```python
from build123d import *

# Parameters (mm, degrees)
EXTRUDE1_DEPTH     = 3.81
EXTRUDE2_DEPTH     = 0.508
CUT_EXTRUDE2_DEPTH = 15.094711526
EXTRUDE3_DEPTH     = 3.048
EXTRUDE4_REACH     = 14.678
SKETCH9_W          = 3.045663376
SKETCH9_H          = 0.1905
SKETCH11_R         = 2.286
CUT_EXTRUDE3_DEPTH = 13.677755519
SKETCH12_R         = 3.175
CUT_EXTRUDE4_DEPTH = 0.508
SKETCH13_OUTSIDE_W = 29.435
SKETCH13_OUTSIDE_H = 14.576
SKETCH13_OUTSIDE_R = 3.81
CUT_EXTRUDE5_DEPTH = 15.094711526
CUT_EXTRUDE7_START = 6.096
CUT_EXTRUDE7_DEPTH = 6.096


with BuildPart() as part:
    # Sketch1 → Extrude1 (new body)
    with BuildSketch(Plane(origin=(0, 0, 0), x_dir=(1, 0, 0), z_dir=(0, 1, 0))):
        with BuildLine():
            Line((-8.001, 3.556), (0, 3.556))
            ThreePointArc((0, 3.556), (3.556, 0), (0, -3.556))
            Line((0, -3.556), (-8.001, -3.556))
            ThreePointArc((-8.001, -3.556), (-11.557, 0), (-8.001, 3.556))
        make_face()
    extrude(amount=EXTRUDE1_DEPTH)

    # Sketch4 → Extrude2 (add)
    with BuildSketch(Plane.XY.offset(3.556)):
        with BuildLine():
            Line((0, 0), (0, 3.81))
            Line((0, 3.81), (7.112, 3.81))
            ThreePointArc((7.112, 3.81), (9.806076836, 2.694076836), (10.922, 0))
            Line((10.922, 0), (7.112, 0))
            Line((7.112, 0), (0, 0))
        make_face()
    extrude2 = extrude(amount=-EXTRUDE2_DEPTH)

    # Sketch6 → Cut-Extrude2 (cut, through all)
    with BuildSketch(Plane.XY.offset(3.556)):
        with BuildLine():
            Line((6.35, 2.032), (6.35, 1.016))
            ThreePointArc((6.35, 1.016), (6.275605122, 0.836394878), (6.096, 0.762))
            Line((6.096, 0.762), (5.08, 0.762))
            ThreePointArc((5.08, 0.762), (4.900394878, 0.687605122), (4.826, 0.508))
            Line((4.826, 0.508), (4.826, -0.508))
            ThreePointArc((4.826, -0.508), (4.900394878, -0.687605122), (5.08, -0.762))
            Line((5.08, -0.762), (6.096, -0.762))
            ThreePointArc((6.096, -0.762), (6.275605122, -0.836394878), (6.35, -1.016))
            Line((6.35, -1.016), (6.35, -2.032))
            ThreePointArc((6.35, -2.032), (6.424394878, -2.211605122), (6.604, -2.286))
            Line((6.604, -2.286), (7.62, -2.286))
            ThreePointArc((7.62, -2.286), (7.799605122, -2.211605122), (7.874, -2.032))
            Line((7.874, -2.032), (7.874, -1.016))
            ThreePointArc((7.874, -1.016), (7.948394878, -0.836394878), (8.128, -0.762))
            Line((8.128, -0.762), (9.144, -0.762))
            ThreePointArc((9.144, -0.762), (9.323605122, -0.687605122), (9.398, -0.508))
            Line((9.398, -0.508), (9.398, 0.508))
            ThreePointArc((9.398, 0.508), (9.323605122, 0.687605122), (9.144, 0.762))
            Line((9.144, 0.762), (8.128, 0.762))
            ThreePointArc((8.128, 0.762), (7.948394878, 0.836394878), (7.874, 1.016))
            Line((7.874, 1.016), (7.874, 2.032))
            ThreePointArc((7.874, 2.032), (7.799605122, 2.211605122), (7.62, 2.286))
            Line((7.62, 2.286), (6.604, 2.286))
            ThreePointArc((6.604, 2.286), (6.424394878, 2.211605122), (6.35, 2.032))
        make_face()
    cut_extrude2 = extrude(amount=-CUT_EXTRUDE2_DEPTH, mode=Mode.SUBTRACT)

    # Sketch8 → Extrude3 (add)
    with BuildSketch(Plane(origin=(0, 0, 3.048), x_dir=(-1, 0, 0), z_dir=(0, 0, -1))):
        with BuildLine():
            Line((-10.287, 0), (-9.906, 0))
            ThreePointArc((-9.906, 0), (-9.218056742, 1.836017701), (-7.493, 2.767900829))
            Line((-7.493, 2.767900829), (-7.493, 3.152057106))
            ThreePointArc((-7.493, 3.152057106), (-9.487952441, 2.106056742), (-10.287, 0))
        make_face()
        with BuildLine():
            Line((-4.318, 0), (-3.937, 0))
            ThreePointArc((-3.937, 0), (-4.736047559, 2.106056742), (-6.731, 3.152057106))
            Line((-6.731, 3.152057106), (-6.731, 2.767900829))
            ThreePointArc((-6.731, 2.767900829), (-5.005943258, 1.836017701), (-4.318, 0))
        make_face()
    extrude3 = extrude(amount=EXTRUDE3_DEPTH)

    # Sketch9 → Extrude4 (add, up to next)
    with BuildSketch(Plane(origin=(0, 0, 0), x_dir=(-1, 0, 0), z_dir=(0, 0, -1)), mode=Mode.PRIVATE) as extrude4_sk1:
        with Locations((-2.604668312, 0.09525)):
            Rectangle(SKETCH9_W, SKETCH9_H)
    extrude4_tool1 = extrude(extrude4_sk1.sketch, amount=-EXTRUDE4_REACH, mode=Mode.PRIVATE) - part.part
    extrude4 = extrude4_tool1.solids().sort_by_distance((2.604668, 0.09525, 0))[0]
    add(extrude4)

    # Mirror5: Extrude2, Cut-Extrude2, Extrude3, Extrude4 across plane
    add(extrude2.mirror(Plane(origin=(7.112, 0, 0), x_dir=(1, 0, 0), z_dir=(0, 0, -1))))
    add(cut_extrude2.mirror(Plane(origin=(7.112, 0, 0), x_dir=(1, 0, 0), z_dir=(0, 0, -1))), mode=Mode.SUBTRACT)
    add(extrude3.mirror(Plane(origin=(7.112, 0, 0), x_dir=(1, 0, 0), z_dir=(0, 0, -1))))
    add(extrude4.mirror(Plane(origin=(7.112, 0, 0), x_dir=(1, 0, 0), z_dir=(0, 0, -1))))

    # Sketch11 → Cut-Extrude3 (cut, through all)
    with BuildSketch(Plane(origin=(0, 3.81, 0), x_dir=(1, 0, 0), z_dir=(0, 1, 0))):
        with Locations(Location((0, 0, 0), (0, 0, 270))):
            Circle(SKETCH11_R)
        with Locations(Location((-8.001, 0, 0), (0, 0, 270))):
            Circle(SKETCH11_R)
    extrude(amount=-CUT_EXTRUDE3_DEPTH, mode=Mode.SUBTRACT)

    # Sketch12 → Cut-Extrude4 (cut)
    with BuildSketch(Plane(origin=(0, 3.81, 0), x_dir=(1, 0, 0), z_dir=(0, 1, 0))):
        with Locations(Location((0, 0, 0), (0, 0, 270))):
            Circle(SKETCH12_R)
        with Locations(Location((-8.001, 0, 0), (0, 0, 270))):
            Circle(SKETCH12_R)
    extrude(amount=-CUT_EXTRUDE4_DEPTH, mode=Mode.SUBTRACT)

    # Mirror6: part across face


with BuildPart() as part_1:
    add(part.part)
    add(part.part.mirror(Plane(origin=(-2.880961452, 0, 0), x_dir=(0, 0, 1), z_dir=(0, -1, 0))))

    # Sketch13 outside → Cut-Extrude5 (cut, through all)
    with BuildSketch(Plane.XY.offset(3.556)):
        with Locations((-0.3175, 0)):
            Rectangle(SKETCH13_OUTSIDE_W, SKETCH13_OUTSIDE_H)
        with Locations((7.112, 0)):
            Circle(SKETCH13_OUTSIDE_R, mode=Mode.SUBTRACT)
    extrude(amount=-CUT_EXTRUDE5_DEPTH, mode=Mode.SUBTRACT)

    # Sketch15 → Cut-Extrude7 (cut)
    with BuildSketch(Plane.XY.offset(-3.048).offset(CUT_EXTRUDE7_START)):
        with BuildLine():
            Line((4.158713877, 2.407114678), (5.041631935, 2.407114678))
            ThreePointArc((5.041631935, 2.407114678), (3.937, 0), (5.041631935, -2.407114678))
            Line((5.041631935, -2.407114678), (4.158713877, -2.407114678))
            ThreePointArc((4.158713877, -2.407114678), (3.302, 0), (4.158713877, 2.407114678))
        make_face()
    extrude(amount=-CUT_EXTRUDE7_DEPTH, mode=Mode.SUBTRACT)


solid = part_1.part
```
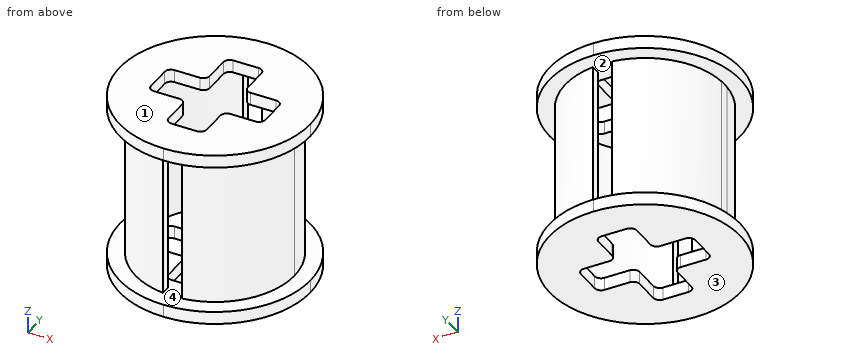
Part model, mm, in its own coordinate system. Face numbers are marked on the shaded views. A direction names the side the tool comes from. Round coordinates to 2 decimals unless told otherwise and drop trailing zeros. Order: outer loops, then holes, each group sorted by start corner. A loop starts at its lowest first (then second) coordinate and runs counter-clockwise, first axis right, second up. Notation, with made-up numbers: M 52.5,73 L 98.5,73 A29 cw 98.5,107 Z; hole C 57.5,27.25 d4. An arc over 180 degrees is marked long. Put each result on its own line as item: value. Start each with the question number.
1. Two-plate mould, pull along Y, no slides. Class the marked faces 1 and 2: +Y half, -Y half, draft (parallel to the pull), parting line (faces both ways), or undercut.
2. Slice it at C-C on y = -1.5. List the corners of the cut face in (x, z), then the cut area to 3 significant figures.
3. Drop flat-ended pins along their axis: pin 1 (1.5 mm diameter, centred on y = 2, z = 0, fed in from -X); pin 2 (4 mm diameter, centred on y = 0.5, z = 0.5, fed in from +X); pin 3 (1 mm diameter, centred on y = -2.5, z = -2, fed in from -X). Give the stop position or say it passes through.
4. Tool access for the marked faces 3 and 4: list every direction of +Z, -Z, +X, -X, +Y, -Y with a clear straight run to the whole face (end or side of a thin tool).
5. Slice it at B-B on x = 8.75. List the corners of the cut face in (y, z).
6. Drill centre lines: probe 1 along Z at (x, y) = (6.75, -2.5); probe 2 along Y at (x, z) = (9, 0.75); probe 3 along X at (y, z) = (2, -0.5). Where is each one in solid material? Low to high. Write a range as [from, to].
7. Slice it at D-D on y = -3. List the corners of the cut face in (x, z), then the cut area to 3 significant figures.
Findings:
1. face 1: draft
1. face 2: undercut
2. outline: M 3.61,-3.56 L 6.35,-3.56 L 6.35,-3.05 L 4.75,-3.05 L 4.75,3.05 L 6.35,3.05 L 6.35,3.56 L 3.61,3.56 L 3.61,3.05 L 4.31,3.05 L 4.31,-3.05 L 3.61,-3.05 Z; M 7.87,-3.56 L 10.61,-3.56 L 10.61,-3.05 L 9.91,-3.05 L 9.91,3.05 L 10.61,3.05 L 10.61,3.56 L 7.87,3.56 L 7.87,3.05 L 9.47,3.05 L 9.47,-3.05 L 7.87,-3.05 Z
2. area: 10.9 mm2
3. pin 1: x = 4.19
3. pin 2: x = 10.29
3. pin 3: x = 4.65
4. face 3: -Z, +X, -X, +Y, -Y
4. face 4: none
5. outline: M -3.44,-3.56 L -0.76,-3.56 L -0.76,-3.05 L -2.26,-3.05 L -2.26,3.05 L -0.76,3.05 L -0.76,3.56 L -3.44,3.56 L -3.44,3.05 L -2.72,3.05 L -2.72,-3.05 L -3.44,-3.05 Z; M 0.76,-3.56 L 3.44,-3.56 L 3.44,-3.05 L 2.72,-3.05 L 2.72,3.05 L 3.44,3.05 L 3.44,3.56 L 0.76,3.56 L 0.76,3.05 L 2.26,3.05 L 2.26,-3.05 L 0.76,-3.05 Z
6. probe 1: [-3.56, -3.05], [3.05, 3.56]
6. probe 2: [-2.55, -2.06], [2.06, 2.55]
6. probe 3: [4.65, 5.16], [9.06, 9.58]
7. outline: M 4.76,-3.56 L 9.46,-3.56 L 9.46,-3.05 L 8.15,-3.05 L 8.15,3.05 L 9.46,3.05 L 9.46,3.56 L 4.76,3.56 L 4.76,3.05 L 6.07,3.05 L 6.07,-3.05 L 4.76,-3.05 Z; hole M 6.73,-3.05 L 7.49,-3.05 L 7.49,3.05 L 6.73,3.05 Z
7. area: 12.8 mm2
